```python
from build123d import *

# Parameters (mm, degrees)
EXTRUDE_1_DEPTH         = 29
HOLE_WIZARD_2_7_2_7_1_D = 2.7
SKETCH_4_R              = 4
EXTRUDE_2_DEPTH         = 2.6
SKETCH_5_R              = 5
EXTRUDE_3_DEPTH         = 0.5
HOLE_WIZARD_M3_1_D      = 2.5
CHAMFER_2_SIZE          = 0.3


with BuildPart() as part:
    # 草图1 → 凸台-拉伸1 (new body)
    with BuildSketch(Plane.XY):
        Polygon((20, 0), (-20, 0), (-20, -9.3), (-17, -9.3), (-17, -3), (17, -3), (17, -9.3), (20, -9.3), align=None)
    extrude(amount=EXTRUDE_1_DEPTH)

    # Ø2.7 (2.7) 直径孔1 (through all)
    with Locations(Plane(origin=(20, 0, 0), x_dir=(0, 0, -1), z_dir=(1, 0, 0))):
        with Locations((-25.5, -6.7), (-3.5, -6.7)):
            Hole(HOLE_WIZARD_2_7_2_7_1_D / 2)

    # 草图4 → 凸台-拉伸2 (add)
    with BuildSketch(Plane(origin=(0, 0, 0), x_dir=(1, 0, 0), z_dir=(0, 1, 0))):
        with Locations(Location((0, -7.5, 0), (0, 0, 90))):
            Circle(SKETCH_4_R)
    extrude(amount=EXTRUDE_2_DEPTH)

    # 草图5 → 凸台-拉伸3 (add)
    with BuildSketch(Plane(origin=(0, 0, 0), x_dir=(1, 0, 0), z_dir=(0, 1, 0))):
        with Locations(Location((0, -7.5, 0), (0, 0, 90))):
            Circle(SKETCH_5_R)
    extrude(amount=EXTRUDE_3_DEPTH)

    # M3 螺纹孔的螺纹孔钻头1 (through all)
    with Locations(Plane(origin=(0, 2.6, 0), x_dir=(1, 0, 0), z_dir=(0, 1, 0))):
        with Locations((0, -7.5)):
            Hole(HOLE_WIZARD_M3_1_D / 2)

    # 倒角2
    chamfer_2_edges = [part.edges().sort_by_distance(p)[0] for p in [
        (0, 2.6, 11.5),
    ]]
    chamfer(chamfer_2_edges, length=CHAMFER_2_SIZE)


solid = part.part
```
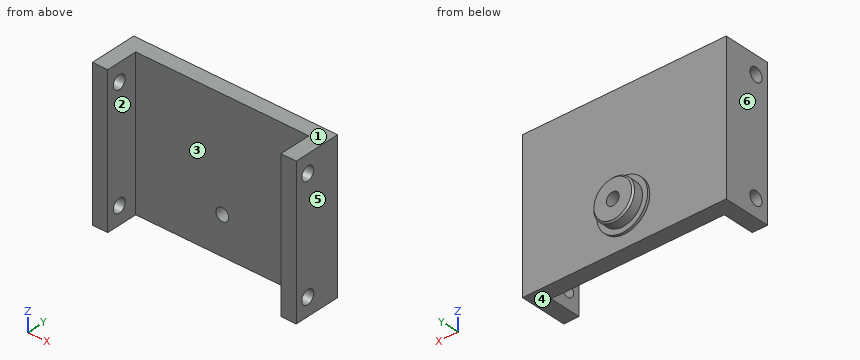
Work out the finished part from the listing and answer in its coordinate system (mm). Face numbers are marked on the shaded views. A direction names the side the tool comes from. Give positions to 0.01 mm unless a question says otherwise; leave off trailing zeros. Order: outer loops, then holes, each group sorted by start corner. A loop starts at its lowest first (then second) coordinate and runs counter-clockwise, first axis right, second up. Notation, with made-up numbers: M 66.25,40.5 L 79.25,40.5 A34 ccw 79.25,77.5 Z; hole C 33,31 d2. An arc over 180 degrees is marked long. Return JSON: item names as keys, results as strings.
1) A tool of negligible diameter and unlimited length cuts with its end or side. For the marked faces 1 and 2, from which of +Z, -Z, +X, -X, +Y, -Y can it reach the whole face along a straight path? Write none if from no direction.
Resolved:
{"face 1": "+Z, +X, -X, +Y, -Y", "face 2": "+Z, -Z, -Y"}
2) Section A-A, the plane y = -6.7 is taken. Write down the section's boundary in (x, z).
Resolved:
{"outline": "M -20,0 L -17,0 L -17,2.15 L -20,2.15 Z; M -20,4.85 L -17,4.85 L -17,24.15 L -20,24.15 Z; M -20,26.85 L -17,26.85 L -17,29 L -20,29 Z; M 17,0 L 20,0 L 20,2.15 L 17,2.15 Z; M 17,4.85 L 20,4.85 L 20,24.15 L 17,24.15 Z; M 17,26.85 L 20,26.85 L 20,29 L 17,29 Z"}
3) Each of these flat-tipped pins is pushed along its axis until it touches: pin 1 (14.5 mm diameter, centred on x = 7.5, z = 8, fed in from -Y); pin 2 (1.5 mm diameter, centred on x = -15.5, z = 8, fed in from +Y). Where does it stop, or does it pass through?
Resolved:
{"pin 1": "y = -3", "pin 2": "y = 0"}
4) Straight lines are drawn through the part: line 1 along X through (y, z) = (-4.5, 12); line 2 along Y through (x, z) = (18, 14.25); line 3 along Y through (x, z) = (-16, 5.5). For each, find the intervals that lie inside material, in ascending order. Write a range as [from, to].
Resolved:
{"line 1": "[-20, -17], [17, 20]", "line 2": "[-9.3, 0]", "line 3": "[-3, 0]"}
5) Section D-D, the plane z = 7.5 is taken. Write down the section's boundary in (x, y), plus the area to 3 significant figures.
Resolved:
{"outline": "M -20,-9.3 L -17,-9.3 L -17,-3 L -1.25,-3 L -1.25,2.6 L -3.7,2.6 L -4,2.3 L -4,0.5 L -5,0.5 L -5,0 L -20,0 Z; M 1.25,-3 L 17,-3 L 17,-9.3 L 20,-9.3 L 20,0 L 5,0 L 5,0.5 L 4,0.5 L 4,2.3 L 3.7,2.6 L 1.25,2.6 Z", "area": "166 mm^2"}
6) For a pull along X with two mould halves and no side action, classify the marked faces 3, 4, 5 and 6 as +X half, -X half, draft (parallel to the pull), parting line (faces both ways), or undercut.
Resolved:
{"face 3": "undercut", "face 4": "draft", "face 5": "+X half", "face 6": "-X half"}
7) Section B-B, the plane z = 25.5 is taken. Write down the section's boundary in (x, y), plus the area to 3 significant figures.
Resolved:
{"outline": "M -20,-9.3 L -17,-9.3 L -17,-8.05 L -20,-8.05 Z; M -20,-5.35 L -17,-5.35 L -17,-3 L 17,-3 L 17,-5.35 L 20,-5.35 L 20,0 L -20,0 Z; M 17,-9.3 L 20,-9.3 L 20,-8.05 L 17,-8.05 Z", "area": "142 mm^2"}
8) Section C-C, the plane x = 0 is taken. Write down the section's boundary in (y, z).
Resolved:
{"outline": "M -3,0 L 0,0 L 0,2.5 L 0.5,2.5 L 0.5,3.5 L 2.3,3.5 L 2.6,3.8 L 2.6,6.25 L -3,6.25 Z; M -3,8.75 L 2.6,8.75 L 2.6,11.2 L 2.3,11.5 L 0.5,11.5 L 0.5,12.5 L 0,12.5 L 0,29 L -3,29 Z"}
